Check sheet for the drawn part. Datum: minimum x, y, z corner. Units: mm. A direction names the side the tool comes from. Round coordinates to 2 decimals unless told otherwise and drop trailing zeros. Loops run counter-clockwise (first coordinate to the right, second up) from the corner with the lowest first, then second, coordinate; pieces in that order, holes last. Notation, with made-up numbers: (-6, 51) -> (12, 51) arc R30 cw to (12, 82) -> close; hole circle Ø4 at (64.25, -25.75). An arc over 180 degrees is marked (long way). Return JSON: item names as keys, results as strings.
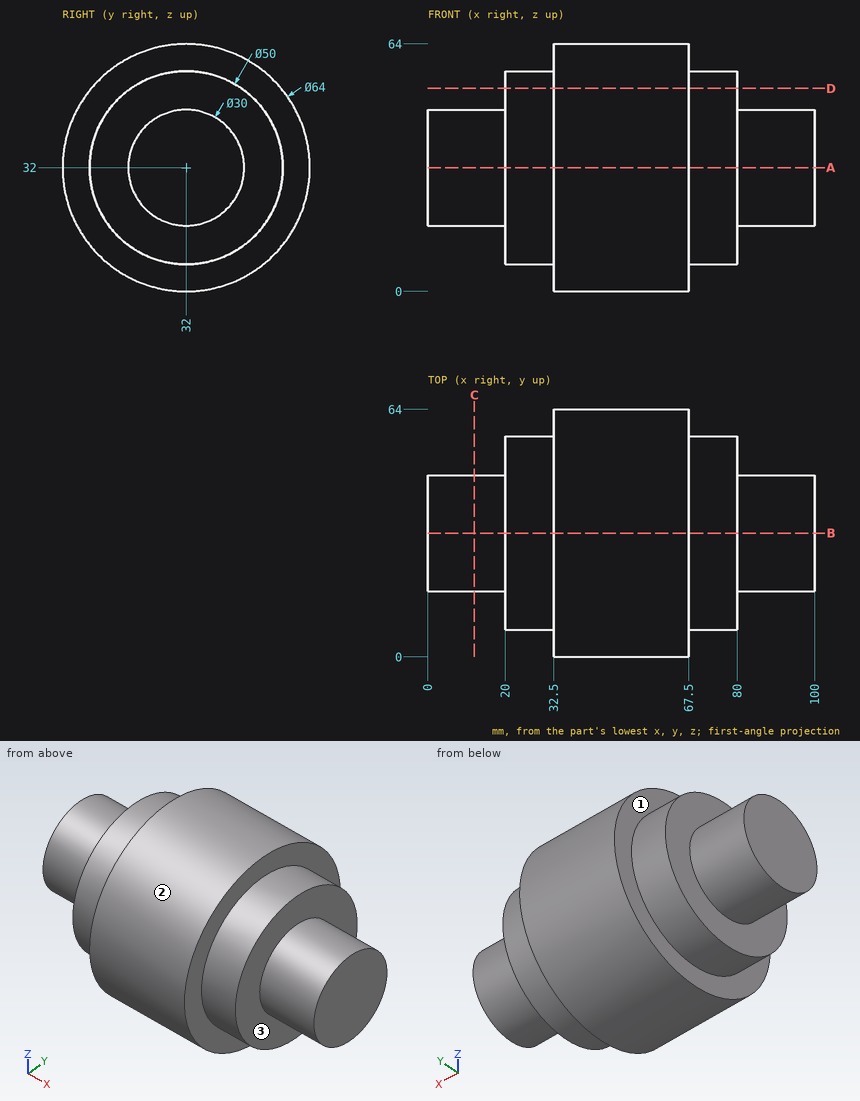
Q1. Section check A-A (z = 32). Record the boundary of the cut face in (x, y), then the cut area to 3 significant figures.
Results list:
{"outline": "(0, 17) -> (20, 17) -> (20, 7) -> (32.5, 7) -> (32.5, 0) -> (67.5, 0) -> (67.5, 7) -> (80, 7) -> (80, 17) -> (100, 17) -> (100, 47) -> (80, 47) -> (80, 57) -> (67.5, 57) -> (67.5, 64) -> (32.5, 64) -> (32.5, 57) -> (20, 57) -> (20, 47) -> (0, 47) -> close", "area": "4,690 mm^2"}
Q2. Section check C-C (x = 12). Record the boundary of the cut face in (y, z), then the cut area to 3 significant figures.
Results list:
{"outline": "circle Ø30 at (32, 32)", "area": "707 mm^2"}
Q3. Go/stop test with flat-tipped pins: pin 1 (10 mm diameter, centred on x = 37, z = 36, fed in from -Y); pin 2 (4 mm diameter, centred on x = 27.5, z = 16.5, fed in from -Y); pin 3 (12 mm diameter, centred on x = 22, y = 36.5, fed in from +Z). Record where each tip stops, or that it passes through.
Results list:
{"pin 1": "y = 0", "pin 2": "y = 10.96", "pin 3": "z = 57"}
Q4. Material ranges on line 1 (Y direction, x = 65.5, z = 32); line 2 (X direction, y = 54, z = 39); line 3 (X direction, y = 49.5, z = 58), recorded low to high.
Results list:
{"line 1": "0 to 64", "line 2": "20 to 80", "line 3": "32.5 to 67.5"}
Q5. Tool access check on the marked faces 1, 2 and 3. Record the directions out of +Z, -Z, +X, -X, +Y, -Y that give a thin tool (end or side, any length) a straight path to the whole face; none if there is none.
Results list:
{"face 1": "-X", "face 2": "+X, -X", "face 3": "+X"}
Q6. Section check D-D (z = 52.5). Record the boundary of the cut face in (x, y).
Results list:
{"outline": "(20, 17.69) -> (32.5, 17.69) -> (32.5, 7.43) -> (67.5, 7.43) -> (67.5, 17.69) -> (80, 17.69) -> (80, 46.31) -> (67.5, 46.31) -> (67.5, 56.57) -> (32.5, 56.57) -> (32.5, 46.31) -> (20, 46.31) -> close"}
